from build123d import *

# Parameters (mm, degrees)
SKETCH_W     = 50
SKETCH_H     = 8
SKETCH_R     = 1.6
PAD_DEPTH    = 3
SKETCH001_W  = 6
SKETCH001_H  = 2
PAD001_DEPTH = 8
SKETCH002_R  = 1.6
POCKET_DEPTH = 5


with BuildPart() as part:
    # Sketch → Pad (new body)
    with BuildSketch(Plane.XY):
        with Locations((-25, 4)):
            Rectangle(SKETCH_W, SKETCH_H)
        with Locations((-43, 5)):
            Circle(SKETCH_R, mode=Mode.SUBTRACT)
        with Locations((-7, 5)):
            Circle(SKETCH_R, mode=Mode.SUBTRACT)
    extrude(amount=PAD_DEPTH)

    # Sketch001 (on Face8 of Pad) → Pad001 (join)
    with BuildSketch(Plane.XY.offset(3)):
        with Locations((-47, 1)):
            Rectangle(SKETCH001_W, SKETCH001_H)
        with Locations((-3, 1)):
            Rectangle(SKETCH001_W, SKETCH001_H)
    extrude(amount=PAD001_DEPTH)

    # Sketch002 (on Face1 of Pad001) → Pocket (cut)
    with BuildSketch(Plane.XZ):
        with Locations((-47, 8.5)):
            Circle(SKETCH002_R)
        with Locations((-3, 8.5)):
            Circle(SKETCH002_R)
    extrude(amount=-POCKET_DEPTH, mode=Mode.SUBTRACT)


solid = part.part
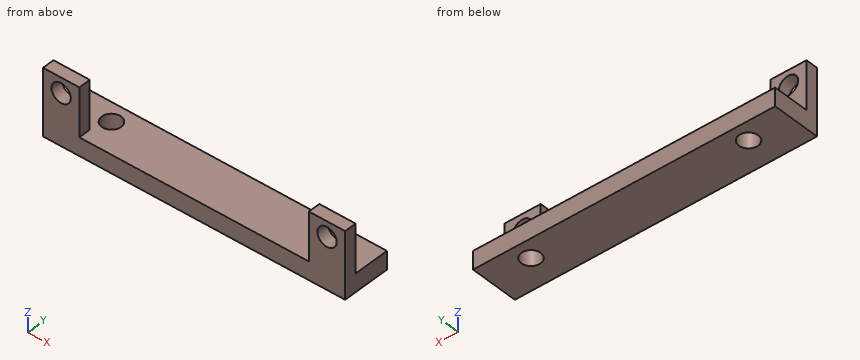
Source: CAD feature listing. Evaluate the final solid. Frame: model axes, mm. Coordinates: 2 decimals unless noted, no trailing zeros. Order: outer loops, then holes, each group sorted by start corner. A loop starts at its lowest first (then second) coordinate and runs counter-clockwise, first axis right, second up. Notation, with made-up numbers: M 65.25,71 L 111.25,71 A13 ccw 111.25,94 Z; hole C 1.5,8.5 d3. An arc over 180 degrees is marked long. Write each question's results on one line, items separated by ' | '. Start each with the question number.
1. Section A-A, the plane z = 4.5. Return the cut outline in (x, y), then the cut area to 3 significant figures.
2. Pin query (flat end, axial travel): pin 1 (6.5 mm diameter, centred on x = -2, z = 7, fed in from +Y); pin 2 (1.9 mm diameter, centred on x = -43, y = 5, fed in from -Z); pin 3 (4 mm diameter, centred on x = -27.5, y = 1.5, fed in from +Z). Return the tip coordinate at first contact, or that it passes through.
3. Section B-B, the plane x = -43. Return the cut outline in (y, z), then the cut area to 3 significant figures.
4. Section D-D, the plane y = 1.5. Return the cut outline in (x, z).
5. Section C-C, the plane y = 5. Return the cut outline in (x, z).
6. Material intervals for L1, parallel to Z at x = -3, y = 0.5; L2, parallel to Y at x = -7, z = 1.85; L3, parallel to Z at x = -10.5, y = 7.25, sorted ascending.
Solution:
1) outline: M -50,0 L -44,0 L -44,2 L -50,2 Z; M -6,0 L 0,0 L 0,2 L -6,2 Z | area: 24.0 mm²
2) pin 1: y = 2 | pin 2: through | pin 3: z = 3
3) outline: M 0,0 L 3.4,0 L 3.4,3 L 0,3 Z; M 6.6,0 L 8,0 L 8,3 L 6.6,3 Z | area: 14.4 mm²
4) outline: M -50,0 L 0,0 L 0,11 L -6,11 L -6,3 L -44,3 L -44,11 L -50,11 Z; hole C -47,8.5 d3.2; hole C -3,8.5 d3.2
5) outline: M -50,0 L -44.6,0 L -44.6,3 L -50,3 Z; M -41.4,0 L -8.6,0 L -8.6,3 L -41.4,3 Z; M -5.4,0 L 0,0 L 0,3 L -5.4,3 Z
6) L1: 0 to 6.9, 10.1 to 11 | L2: 0 to 3.4, 6.6 to 8 | L3: 0 to 3
